from build123d import *

# Parameters (mm, degrees)
F0_R     = 7.375
F1_DEPTH = 18
F4_R     = 5.207
F5_DEPTH = 14.751
F6_D     = 7.9375


with BuildPart() as f1:
    # F0 (on Top) → F1 (new body)
    with BuildSketch(Plane.XY):
        Circle(F0_R)
    extrude(amount=F1_DEPTH)

    # F4 (on plane+point) → F5 (cut, through all)
    with BuildSketch(Plane.YZ.offset(-7.375)):
        with Locations((0, 11.65)):
            Circle(F4_R)
    extrude(amount=F5_DEPTH, mode=Mode.SUBTRACT)

    # F6 (through all)
    with Locations(Plane.XY.offset(18)):
        with Locations((0, 0)):
            Hole(F6_D / 2)


solid = f1.part
Geometry: final body of the model. Coordinates: model frame, mm. Coordinates: 2 decimals unless noted, no trailing zeros. Order: outer loops, then holes, each group sorted by start corner. A loop starts at its lowest first (then second) coordinate and runs counter-clockwise, first axis right, second up.
(1) Section query A-A (x = 0). Return the cut outline in (y, z) (3 decimals), plus the area to 3 significant figures.
(2) First-contact query: pin 1 (6 mm diameter, centred on y = 3.5, z = 10, fed in from +X); pin 2 (5 mm diameter, centred on y = 4.5, z = 11, fed in from +X); pin 3 (4 mm diameter, centred on x = -2.5, z = 14, fed in from -Y). Flat tips, straight axial feed; report the tip coordinate or a pass-through.
(3) Section query B-B (y = -1.75). Return the cut outline in (x, z).
(4) Material intervals for probe 1 along X at (y, z) = (0, 2.5) (3 decimals); probe 2 along Y at (x, z) = (1.25, 12.5), sorted ascending.
(5) Draft query along Y for faces 1 (the face through (-3.666, -1.52, 16.821)), 2 (the face through (3.149, -2.415, 4.082)), 3 (the face through (3, -3, 18)), 4 (the face through (3.96, 6.22, 8.87)). Return one class per face: pulls with the +Y half, pulls with the -Y half, needs draft (parallel to the pull), parting line crosses it, or undercut.
Solution:
1. outline: (-7.375, 0) - (-3.969, 0) - (-3.969, 8.279) arc R5.207 cw to (-3.969, 15.021) - (-3.969, 18) - (-7.375, 18) - close; (3.969, 0) - (7.375, 0) - (7.375, 18) - (3.969, 18) - (3.969, 15.021) arc R5.207 cw to (3.969, 8.279) - close
1. area: 111 mm2
2. pin 1: stops at x = 6.9
2. pin 2: stops at x = 6.09
2. pin 3: stops at y = -7.36
3. outline: (-7.16, 0) - (-3.56, 0) - (-3.56, 6.75) - (-7.16, 6.75) - close; (-7.16, 16.55) - (-3.56, 16.55) - (-3.56, 18) - (-7.16, 18) - close; (3.56, 0) - (7.16, 0) - (7.16, 6.75) - (3.56, 6.75) - close; (3.56, 16.55) - (7.16, 16.55) - (7.16, 18) - (3.56, 18) - close
4. probe 1: x = -7.375 to -3.969, 3.969 to 7.375
4. probe 2: y = -7.27 to -5.14, 5.14 to 7.27
5. face 1: undercut
5. face 2: undercut
5. face 3: needs draft
5. face 4: parting line crosses it
